Here's the drawing with two shaded views (mm, measured from the low corner). I have some questions. A direction names the side the tool comes from. Round coordinates to 2 decimals unless told otherwise and drop trailing zeros. Loops run counter-clockwise (first coordinate to the right, second up) from the corner with the lowest first, then second, coordinate; pieces in that order, holes last. Notation, with made-up numbers: M 7.25,84.25 L 41.25,84.25 A16 ccw 41.25,88.25 Z; hole C 66.25,-18 d1. An arc over 180 degrees is marked long. Answer as a JSON object with one key per item and string values.
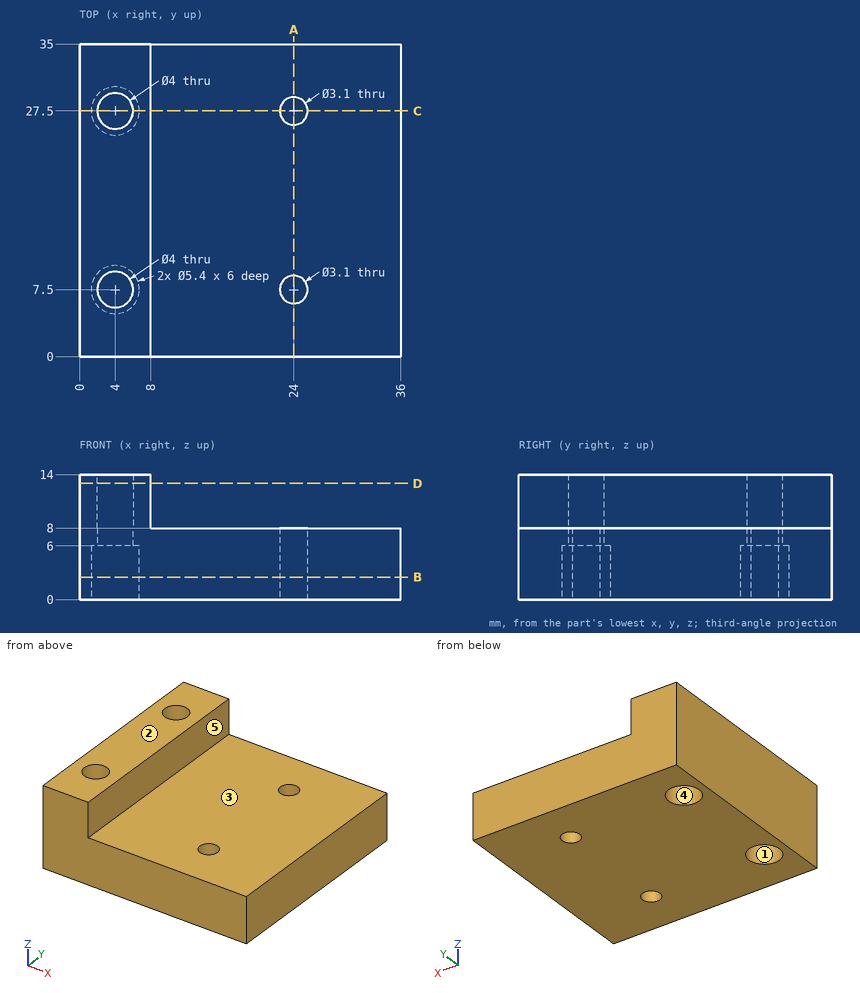
Item 1: I want a section at A-A on x = 24. List the corners of the cut face in (y, z) for me, plus the area to 3 significant figures.
Solution:
{"outline": "M 0,0 L 5.95,0 L 5.95,8 L 0,8 Z; M 9.05,0 L 25.95,0 L 25.95,8 L 9.05,8 Z; M 29.05,0 L 35,0 L 35,8 L 29.05,8 Z", "area": "230 mm2"}
Item 2: We'd pull the mould along X, two halves only. Please class the marked faces 3, 4 and 5: +X half, -X half, draft (parallel to the pull), parting line (faces both ways), or undercut.
Solution:
{"face 3": "draft", "face 4": "undercut", "face 5": "+X half"}
Item 3: I want a section at C-C on y = 27.5. List the corners of the cut face in (x, z) for me.
Solution:
{"outline": "M 0,0 L 1.3,0 L 1.3,6 L 2,6 L 2,14 L 0,14 Z; M 6,6 L 6.7,6 L 6.7,0 L 22.45,0 L 22.45,8 L 8,8 L 8,14 L 6,14 Z; M 25.55,0 L 36,0 L 36,8 L 25.55,8 Z"}
Item 4: I want a section at D-D on z = 13. List the corners of the cut face in (x, y) for me, plus the area to 3 significant figures.
Solution:
{"outline": "M 0,0 L 8,0 L 8,35 L 0,35 Z; hole C 4,7.5 d4; hole C 4,27.5 d4", "area": "255 mm2"}
Item 5: For P1, Ø6, axis at y = 13, z = 10, coming from the +X side; P2, Ø10, axis at x = 16.5, y = 7.5, coming from the +Z side; P3, Ø3, axis at x = 4, y = 27.5, coming from the +Z side, each with a flat end and sliding along its axis, tell me the tip position at first contact or that it passes through.
Solution:
{"P1": "stops at x = 36", "P2": "stops at z = 8", "P3": "passes through"}
Item 6: For the marked faces 1 and 2, which set-ups out of +Z, -Z, +X, -X, +Y, -Y let a thin tool reach every point of the face, with its end or its side?
Solution:
{"face 1": "-Z", "face 2": "+Z, +X, -X, +Y, -Y"}
Item 7: I want a section at B-B on z = 2.5. List the corners of the cut face in (x, y) for me.
Solution:
{"outline": "M 0,0 L 36,0 L 36,35 L 0,35 Z; hole C 4,7.5 d5.4; hole C 4,27.5 d5.4; hole C 24,7.5 d3.1; hole C 24,27.5 d3.1"}
Item 8: If I drill on L1, parallel to Y at x = 4, z = 7.45; L2, parallel to Y at x = 4, z = 1.7; L3, parallel to X at y = 6.5, z = 2, over which ranges is the centre line in solid material (lowest first)? Write a range as from..to.
Solution:
{"L1": "y = 0..5.5, 9.5..25.5, 29.5..35", "L2": "y = 0..4.8, 10.2..24.8, 30.2..35", "L3": "x = 0..1.49, 6.51..22.82, 25.18..36"}
